Read the model definition and answer for the solid it produces. Units are mm, in the model's axes. A direction names the side the tool comes from. Coordinates: 2 decimals unless noted, no trailing zeros. Loops run counter-clockwise (first coordinate to the right, second up) from the corner with the lowest first, then second, coordinate; pieces in that order, holes last.
Q1. Straight lines are drawn through the part: line 1 (Y direction, x = 2, z = 15); line 2 (Z direction, x = 1.5, y = 5.5); line 3 (Y direction, x = 0, z = -19). For each, find the intervals that lie inside material, in ascending order.
Q2. Section C-C (z = 15) is taken. Give the vertices of the cut face in (x, y), then the cut area to 3 significant figures.
Q3. Flat-ended cylindrical pins translate along their axes: P1, Ø8, axis at x = -24, z = 35, coming from the +Y side; P2, Ø6, axis at y = 10, z = -15, coming from the +X side; P3, Ø20, axis at y = 4.5, z = 10.5, coming from the -X side. Find the tip coordinate at first contact, or state that the pin passes through.
Q4. Section A-A (x = -18) is taken. Give the vertices of the cut face in (y, z).
Q5. The mould has two halves that part along X. Classify faces 1 (the face through (-27, -15, -33)), 2 (the face through (-21, -10, 0)), 3 (the face through (-0.651, -5.043, 0.525)): pulls with the +X half, pulls with the -X half, needs draft (parallel to the pull), parting line crosses it, or undercut.
Q6. Section D-D (x = 0) is taken. Give the vertices of the cut face in (y, z).
Q7. Section B-B (y = -7) is taken. Give the vertices of the cut face in (x, z), then the cut area to 3 significant figures.
Q8. Which of the six approach directions +Z, -Z, +X, -X, +Y, -Y give full straight-line access (tool end or side, diameter ignored) to faces 4 (the face through (-20, -15, -25.5)), 5 (the face through (-25.99, -15.07, 27.35)), 6 (the face through (-27, -15, 32)), 7 (the face through (-21, -10, -32))?
from build123d import *

# Parameters (mm, degrees)
SKETCH1_W             = 30
SKETCH1_H             = 75
MAIN_BLOCK_DEPTH      = 20
FRAME_HOLE_REACH      = 81.057
SKETCH2_R             = 5
EM_ROD_HOLES_REACH    = 54.022
EM_ROD_HOLES_SKETCH_R = 4.9
SKETCH4_W             = 12
SKETCH4_H             = 75
BOSS_EXTRUDE1_DEPTH   = 10
CUT_EXTRUDE1_DEPTH    = 62.116691664


with BuildPart() as part:
    # Sketch1 → Main Block (new, symmetric)
    with BuildSketch(Plane(origin=(0, 0, 0), x_dir=(1, 0, 0), z_dir=(0, 1, 0))):
        Rectangle(SKETCH1_W, SKETCH1_H)
    extrude(amount=MAIN_BLOCK_DEPTH, both=True)

    # Sketch2 → Frame Hole (cut, up to next)
    with BuildSketch(Plane.XY.offset(37.5), mode=Mode.PRIVATE) as frame_hole_sk1:
        with Locations((0, -10)):
            Circle(SKETCH2_R)
    frame_hole_tool1 = extrude(frame_hole_sk1.sketch, amount=-FRAME_HOLE_REACH, mode=Mode.PRIVATE) & part.part
    add(frame_hole_tool1.solids().sort_by_distance((0, -10, 37.5))[0], mode=Mode.SUBTRACT)

    # EM Rod Holes Sketch → EM Rod Holes (cut, up to next)
    with BuildSketch(Plane(origin=(15, 0, 0), x_dir=(0, 0, -1), z_dir=(1, 0, 0)), mode=Mode.PRIVATE) as em_rod_holes_sk1:
        with Locations((-15, 10)):
            Circle(EM_ROD_HOLES_SKETCH_R)
    em_rod_holes_tool1 = extrude(em_rod_holes_sk1.sketch, amount=-EM_ROD_HOLES_REACH, mode=Mode.PRIVATE) & part.part
    # EM Rod Holes Sketch → EM Rod Holes (cut, up to next)
    with BuildSketch(Plane(origin=(15, 0, 0), x_dir=(0, 0, -1), z_dir=(1, 0, 0)), mode=Mode.PRIVATE) as em_rod_holes_sk2:
        with Locations((15, 10)):
            Circle(EM_ROD_HOLES_SKETCH_R)
    em_rod_holes_tool2 = extrude(em_rod_holes_sk2.sketch, amount=-EM_ROD_HOLES_REACH, mode=Mode.PRIVATE) & part.part
    add(em_rod_holes_tool1.solids().sort_by_distance((15, 10, 15))[0], mode=Mode.SUBTRACT)
    add(em_rod_holes_tool2.solids().sort_by_distance((15, 10, -15))[0], mode=Mode.SUBTRACT)

    # Sketch4 → Boss-Extrude1 (add)
    with BuildSketch(Plane.XZ.offset(20)):
        with Locations((-21, 0)):
            Rectangle(SKETCH4_W, SKETCH4_H)
    extrude(amount=-BOSS_EXTRUDE1_DEPTH)

    # Sketch6 → Cut-Extrude1 (cut, symmetric)
    with BuildSketch(Plane.XZ.offset(20)):
        with BuildLine():
            ThreePointArc((-25, 27.3), (-26.004987562, 27.350124379), (-27, 27.5))
            Line((-27, 27.5), (-27, 25.5))
            ThreePointArc((-27, 25.5), (-26.004987562, 25.649875621), (-25, 25.7))
            ThreePointArc((-25, 25.7), (-24.858578644, 25.641421356), (-24.8, 25.5))
            Line((-24.8, 25.5), (-15, 25.5))
            Line((-15, 25.5), (-15, 27.5))
            Line((-15, 27.5), (-24.8, 27.5))
            ThreePointArc((-24.8, 27.5), (-24.858578644, 27.358578644), (-25, 27.3))
        make_face()
    cut_extrude1 = extrude(amount=CUT_EXTRUDE1_DEPTH, both=True, mode=Mode.SUBTRACT)

    # Mirror1: Cut-Extrude1 across plane
    add(cut_extrude1.mirror(Plane.XY), mode=Mode.SUBTRACT)


solid = part.part
Numbers:
1. line 1: y = -20 to -14.58, -5.42 to 5.1, 14.9 to 20
1. line 2: z = -37.5 to -16.94, -13.06 to 13.06, 16.94 to 37.5
1. line 3: y = -20 to -15, -5 to 7.17, 12.83 to 20
2. outline: (-27, -20) - (15, -20) - (15, 5.1) - (-15, 5.1) - (-15, -10) - (-27, -10) - close; (-15, 14.9) - (15, 14.9) - (15, 20) - (-15, 20) - close; hole circle Ø10 at (0, -10)
2. area: 947 mm2
3. P1: stops at y = -10
3. P2: passes through
3. P3: stops at x = -15
4. outline: (-20, -37.5) - (-10, -37.5) - (-10, -27.5) - (-20, -27.5) - close; (-20, -25.5) - (-10, -25.5) - (-10, 25.5) - (-20, 25.5) - close; (-20, 27.5) - (-10, 27.5) - (-10, 37.5) - (-20, 37.5) - close
5. face 1: pulls with the -X half
5. face 2: needs draft
5. face 3: undercut
6. outline: (-20, -37.5) - (-15, -37.5) - (-15, 37.5) - (-20, 37.5) - close; (-5, -37.5) - (20, -37.5) - (20, 37.5) - (-5, 37.5) - close; hole circle Ø9.8 at (10, -15); hole circle Ø9.8 at (10, 15)
7. outline: (-15, -37.5) - (-4, -37.5) - (-4, 37.5) - (-15, 37.5) - close; (4, -37.5) - (15, -37.5) - (15, 37.5) - (4, 37.5) - close
7. area: 1,650 mm2
8. face 4: +Y, -Y
8. face 5: -X, +Y, -Y
8. face 6: +Z, -Z, -X, +Y, -Y
8. face 7: +Z, -Z, -X, +Y
